Autodesk Inventor part; units mm, degrees
ref_plane "YZ Plane" through (0, 0, 0) normal (1, 0, 0) x (0, 1, 0)
ref_plane "XZ Plane" through (0, 0, 0) normal (0, 1, 0) x (-1, 0, 0)
ref_plane "XY Plane" through (0, 0, 0) normal (0, 0, 1) x (1, 0, 0)
sketch "Sketch1" plane through (0, 0, 0) normal (0, 0, 1) x (1, 0, 0)
  line L0 (2, 0) -> (40.67, 0)
  line L1 (42.67, 2) -> (42.67, 40.67)
  line L2 (40.67, 42.67) -> (2, 42.67)
  line L3 (0, 40.67) -> (0, 2)
  line L4 (2, 42.67) -> (0, 40.67)
  line L5 (0, 2) -> (2, 0)
  line L6 (40.67, 0) -> (42.67, 2)
  line L7 (42.67, 40.67) -> (40.67, 42.67)
  circle A0 centre (21.335, 21.335) radius 11.5
  line L8 (5.835, 36.835) -> (36.835, 36.835) construction
  line L9 (36.835, 36.835) -> (36.835, 5.835) construction
  line L10 (36.835, 5.835) -> (5.835, 5.835) construction
  line L11 (5.835, 5.835) -> (5.835, 36.835) construction
  circle A1 centre (5.835, 36.835) radius 1.6
  circle A2 centre (36.835, 36.835) radius 1.6
  circle A3 centre (36.835, 5.835) radius 1.6
  circle A4 centre (5.835, 5.835) radius 1.6
  point P0 (0, 0)
  point P1 (42.67, 42.67)
  point P2 (42.67, 0)
  point P3 (0, 42.67)
  point P4 (42.67, 21.335)
  point P5 (21.335, 42.67)
  point P6 (21.335, 36.835)
  point P7 (36.835, 21.335)
  dimension "d0" = 2
  dimension "d1" = 2
  dimension "d2" = 2
  dimension "d3" = 2
  dimension "d4" = 2
  dimension "d5" = 2
  dimension "d6" = 2
  dimension "d7" = 2
  dimension "d8" = 42.67
  dimension "d9" = 42.67
  dimension "d10" = 23
  dimension "d11" = 31
  dimension "d12" = 31
  dimension "d13" = 3.2
  dimension "d14" = 3.2
  dimension "d15" = 3.2
  dimension "d16" = 3.2
extrude "Extrusion1" add sketch "Sketch1" along normal blind 6.5
properties part number "x_motor_spacer"
Verification items for the finished model (mm, model axes). Coordinates: 2 decimals unless noted, no trailing zeros. Write each loop counter-clockwise with the first axis right and the second up, starting at its lowest first coordinate (ties: lowest second). Pieces come first, ordered by that corner, then holes. Notation, with made-up numbers: (72.25, 47) - (85.25, 47) arc R35 cw to (85.25, 85) - close; hole circle Ø7 at (36, 9.25). An arc over 180 degrees is marked (long way). Answer as a JSON object with one key per item and string values.
(1) Mould release check, pull along X, two halves, no side actions. Record for faces 1 (the flat face through (22, 42.67, 3)), 2 (the flat face through (1, 1, 3)), 3 (the cylindrical face through (32.304, 17.881, 3.204)): pulls with the +X half, pulls with the -X half, needs draft (parallel to the pull), parting line crosses it, or undercut.
Report:
{"face 1": "needs draft", "face 2": "pulls with the -X half", "face 3": "undercut"}
(2) Thickness scan on line 1 along X through (y, z) = (37, 3); line 2 along Y through (x, z) = (37.5, 4.25); line 3 along Y through (x, z) = (5, 0.5). Record the ranges inside material, lowest first.
Report:
{"line 1": "0 to 4.24, 7.43 to 35.24, 38.43 to 42.67", "line 2": "0 to 4.38, 7.29 to 35.38, 38.29 to 42.67", "line 3": "0 to 4.47, 7.2 to 35.47, 38.2 to 42.67"}
(3) Cross-section at B-B on y = 25. Record the cut outline in (x, z).
Report:
{"outline": "(0, 0) - (10.43, 0) - (10.43, 6.5) - (0, 6.5) - close; (32.24, 0) - (42.67, 0) - (42.67, 6.5) - (32.24, 6.5) - close"}
(4) Cross-section at D-D on z = 4.75. Record the cut outline in (x, y) (3 decimals).
Report:
{"outline": "(0, 2) - (2, 0) - (40.67, 0) - (42.67, 2) - (42.67, 40.67) - (40.67, 42.67) - (2, 42.67) - (0, 40.67) - close; hole circle Ø3.2 at (5.835, 5.835); hole circle Ø3.2 at (5.835, 36.835); hole circle Ø23 at (21.335, 21.335); hole circle Ø3.2 at (36.835, 5.835); hole circle Ø3.2 at (36.835, 36.835)"}
(5) Cross-section at C-C on x = 5. Record the cut outline in (y, z), plus the area to 3 significant figures.
Report:
{"outline": "(0, 0) - (4.47, 0) - (4.47, 6.5) - (0, 6.5) - close; (7.2, 0) - (35.47, 0) - (35.47, 6.5) - (7.2, 6.5) - close; (38.2, 0) - (42.67, 0) - (42.67, 6.5) - (38.2, 6.5) - close", "area": "242 mm^2"}
(6) Cross-section at A-A on x = 20.5. Record the cut outline in (y, z).
Report:
{"outline": "(0, 0) - (9.87, 0) - (9.87, 6.5) - (0, 6.5) - close; (32.8, 0) - (42.67, 0) - (42.67, 6.5) - (32.8, 6.5) - close"}
